Source: CAD feature listing. Evaluate the final solid. Frame: model axes, mm. Face numbers are marked on the shaded views. Give positions to 0.01 mm unless a question says otherwise; leave off trailing zeros. Order: outer loops, then holes, each group sorted by start corner. A loop starts at its lowest first (then second) coordinate and runs counter-clockwise, first axis right, second up. Notation, with made-up numbers: (88.25, -15) -> (117.25, -15) arc R28 cw to (117.25, 3) -> close; hole circle Ø10 at (72, 45.25). An arc over 180 degrees is marked (long way). Use one line per item in the form item = value. Start each with the question number.
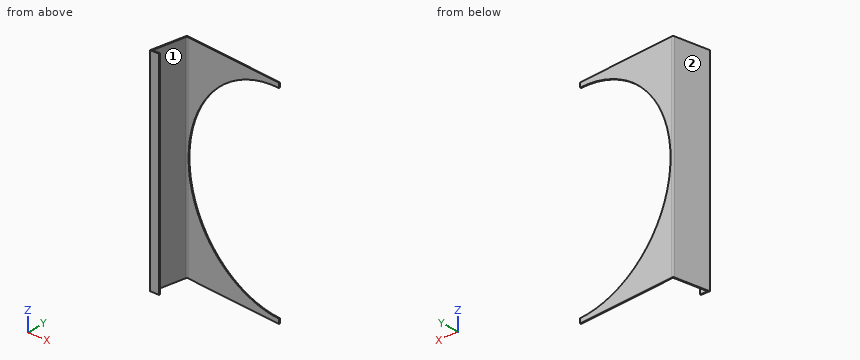
Autodesk Inventor part; units mm, degrees
ref_plane "YZ Plane" through (0, 0, 0) normal (1, 0, 0) x (0, 1, 0)
ref_plane "XZ Plane" through (0, 0, 0) normal (0, 1, 0) x (-1, 0, 0)
ref_plane "XY Plane" through (0, 0, 0) normal (0, 0, 1) x (1, 0, 0)
sketch "Sketch1" plane through (0, 0, 0) normal (0, 0, 1) x (1, 0, 0)
  line L0 (3.739, 2.921) -> (19.8226, 94.1354)
  line L1 (304.8, 66.421) -> (304.8011, 69.342)
  line L2 (304.8011, 69.342) -> (20.634, 99.9646)
  line L3 (17.1671, 97.3593) -> (0, 0)
  line L4 (0, 0) -> (25.4, 0)
  line L5 (25.4, 0) -> (25.4, 2.921)
  line L6 (25.4, 2.921) -> (3.739, 2.921)
  line L7 (23.2893, 96.7408) -> (304.8, 66.421)
  arc A0 (20.634, 99.9646) -> (17.1671, 97.3593) centre (20.2938, 96.8079) ccw
  arc A1 (23.2893, 96.7408) -> (19.8226, 94.1354) centre (22.9493, 93.584) ccw
  point P0 (20.338, 97.0586)
  point P1 (17.6825, 100.2827)
  dimension "d4" = 101.6
  dimension "d12" = 3.175
  dimension "d13" = 25.4
  dimension "d14" = 2.921
  dimension "d15" = 304.8
  dimension "d17" = 80
  dimension "d19" = 2.921
  dimension "d21" = 63.5
  dimension "d24" = 2.921
  dimension "d25" = 93.849
  dimension "d26" = 3.175
extrude "Extrusion1" add sketch "Sketch1" along normal mid plane 584.2
sketch "Sketch2" plane through (0, 0, 0) normal (0, 1, 0) x (-1, 0, 0)
  circle A0 centre (-304.8, 0) radius 279.4
  line L0 (0, -292.1) -> (0, 292.1)
  point P0 (0, 0)
  point P1 (0, 0)
  dimension "d8" = 558.8
  dimension "d9" = 304.8
extrude "Extrusion2" cut sketch "Sketch2" along normal through all
properties part number "CarouselRamp" material "Polycarbonate, Smoke"
1) Cut plane C-C, the plane x = 186. Return the cut outline in (y, z).
2) Cut plane A-A, the plane x = 86. Return the cut outline in (y, z).
3) Material intervals for probe 1 along Z at (x, y) = (246.5, 73.5); probe 2 along X at (y, z) = (60, -130.5); probe 3 along X at (y, z) = (49, -108.5), sorted ascending.
4) Cut plane B-B, the plane z = -76.5. Return the cut outline in (x, y).
5) Cut plane D-D, the plane z = 94. Return the cut outline in (x, y).
6) Pin query (flat end, axial travel): pin 1 (8 mm diameter, centred on y = 12, z = -163, fed in from -X); pin 2 (2.5 mm diameter, centred on y = 2, z = -107, fed in from +X); pin 3 (3 mm diameter, centred on y = 19, z = 94.5, fed in from -X). Return the tip coordinate at first contact, or that it passes through.
7) Draft query along Y for the marked faces 1 and 2. Return one class per face: +Y half, -Y half, draft (parallel to the pull), parting line (faces both ways), or undercut.
Output values:
q1.outline = (79.22, -292.1) -> (82.14, -292.1) -> (82.14, -252.89) -> (79.22, -252.89) -> close; (79.22, 252.89) -> (82.14, 252.89) -> (82.14, 292.1) -> (79.22, 292.1) -> close
q2.outline = (89.99, -292.1) -> (92.92, -292.1) -> (92.92, -173.76) -> (89.99, -173.76) -> close; (89.99, 173.76) -> (92.92, 173.76) -> (92.92, 292.1) -> (89.99, 292.1) -> close
q3.probe_1 = -292.1 to -273.25, 273.25 to 292.1
q3.probe_2 = 10.58 to 13.8
q3.probe_3 = 8.64 to 11.86
q4.outline = (0, 0) -> (25.4, 0) -> (25.4, 2.92) -> (3.74, 2.92) -> (19.82, 94.14) arc R3.17 cw to (23.29, 96.74) -> (36.08, 95.36) -> (36.08, 98.3) -> (20.63, 99.96) arc R3.17 ccw to (17.17, 97.36) -> close
q5.outline = (0, 0) -> (25.4, 0) -> (25.4, 2.92) -> (3.74, 2.92) -> (19.82, 94.14) arc R3.17 cw to (23.29, 96.74) -> (41.69, 94.76) -> (41.69, 97.7) -> (20.63, 99.96) arc R3.17 ccw to (17.17, 97.36) -> close
q6.pin_1 = 1.41
q6.pin_2 = 25.4
q6.pin_3 = 3.09
q7.face_1 = undercut
q7.face_2 = +Y half
